Can you work these out from the model? Positions are in its coordinate system, mm. Face numbers are marked on the shaded views. A direction names the side the tool comes from. Give positions to 0.01 mm unless a question says otherwise; leave off trailing zeros. Write each loop counter-clockwise with the first axis right and the second up, starting at its lowest first coordinate (ties: lowest second). Pieces come first, ordered by that corner, then holes.
1. I'm going to push flat-ended pins straight in: pin 1 (20.5 mm diameter, centred on x = 14, y = 37.5, fed in from +Z); pin 2 (1 mm diameter, centred on x = 29.5, y = 10, fed in from +Z); pin 3 (12.5 mm diameter, centred on x = 16.5, z = 58, fed in from +Y). Where does each tip first touch, or does it pass through?
2. Suppose I cut it at B-B (y = 13). Please give me the cut outline in (x, z), and give its area (3 significant figures).
3. Suppose I cut it at C-C (z = 33.5). Please give me the cut outline in (x, y), and give its area (3 significant figures).
4. If I drill on probe 1 along Y at (x, z) = (36.5, 63); probe 2 along Z at (x, y) = (34.5, 31); probe 3 along Y at (x, z) = (16.5, 33.5), over which ranges is the centre line in solid material (lowest first)?
5. On a 3-axis mill with a long thin cutter (end or side, diameter ignored), from which of +Z, -Z, +X, -X, +Y, -Y can I reach the whole of each face in a straight line? I mean the marked faces 1 and 2. Say none if no direction works.
6. Suppose I cut it at A-A (x = 39). Please give me the cut outline in (y, z).
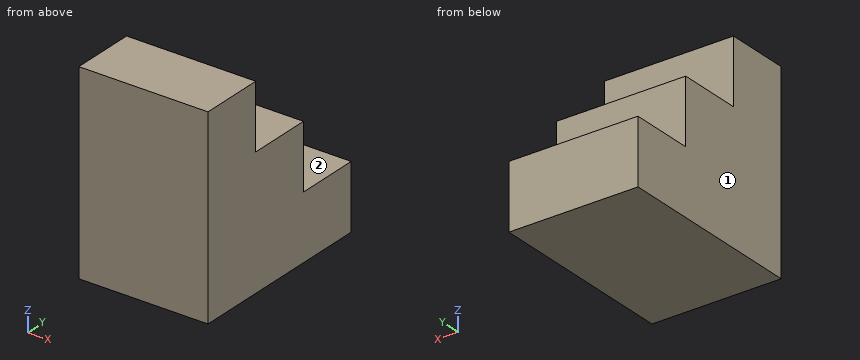
```python
from build123d import *

# Parameters (mm, degrees)
F0_W      = 50.8
F0_H      = 76.2
F1_DEPTH  = 25.4
F2_W      = 50.8
F2_H      = 50.8
F1_FACE_W = 50.8
F1_FACE_H = 76.2
F3_DEPTH  = 25.4
F4_W      = 50.8
F4_H      = 25.4
F5_DEPTH  = 50.8


with BuildPart() as f1:
    # F0 (on Front) → F1 (new body)
    with BuildSketch(Plane.XZ):
        with Locations((25.4, 38.1)):
            Rectangle(F0_W, F0_H)
    extrude(amount=F1_DEPTH)

    # F2 (on Front) + F1_face (on face) → F3 (join)
    with BuildSketch(Plane.XZ):
        with Locations((25.4, 25.4)):
            Rectangle(F2_W, F2_H)
    with BuildSketch(Plane(origin=(25.4, -25.4, 38.1), x_dir=(1, 0, 0), z_dir=(0, -1, 0))):
        Rectangle(F1_FACE_W, F1_FACE_H)
    extrude(amount=-F3_DEPTH)

    # F4 (on Front) → F5 (join)
    with BuildSketch(Plane.XZ):
        with Locations((25.4, 12.7)):
            Rectangle(F4_W, F4_H)
    extrude(amount=-F5_DEPTH)


solid = f1.part
```
Checks:
1. pin 1: stops at z = 25.4
1. pin 2: stops at z = 50.8
1. pin 3: stops at y = 0
2. outline: (0, 0) - (50.8, 0) - (50.8, 50.8) - (0, 50.8) - close
2. area: 2,580 mm2
3. outline: (0, -25.4) - (50.8, -25.4) - (50.8, 25.4) - (0, 25.4) - close
3. area: 2,580 mm2
4. probe 1: y = -25.4 to 0
4. probe 2: z = 0 to 25.4
4. probe 3: y = -25.4 to 25.4
5. face 1: +Z, -Z, -X, +Y, -Y
5. face 2: +Z, +X, -X, +Y
6. outline: (-25.4, 0) - (50.8, 0) - (50.8, 25.4) - (25.4, 25.4) - (25.4, 50.8) - (0, 50.8) - (0, 76.2) - (-25.4, 76.2) - close
